For this review, take the finished solid that the model builds, in its own axes (mm). Face numbers are marked on the shaded views. Give positions to 0.01 mm unless a question says otherwise; leave off trailing zeros.
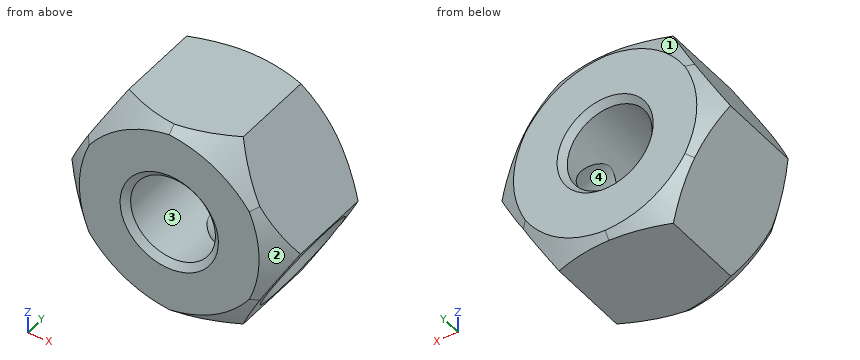
from build123d import *
from OCP.BRepFilletAPI import BRepFilletAPI_MakeChamfer

# Parameters (mm, degrees)
SKETCH1_R           = 1.5
BOSS_EXTRUDE1_DEPTH = 4.5
CHAMFER1_SIZE       = 0.2
CHAMFER1_SIZE2      = 0.238350719
SKETCH2_R           = 1.4
CUT_EXTRUDE1_DEPTH  = 3
CHAMFER2_SIZE       = 0.4
CHAMFER2_SIZE_2     = 0.476701437
FILLET1_R           = 5.5


with BuildPart() as part:
    # Sketch1 → Boss-Extrude1 (new body)
    with BuildSketch(Plane(origin=(0, 0, 0), x_dir=(1, 0, 0), z_dir=(0, 1, 0))):
        Polygon((4.041451884, 0), (2.020725942, 3.5), (-2.020725942, 3.5), (-4.041451884, 0), (-2.020725942, -3.5), (2.020725942, -3.5), align=None)
        with Locations(Location((0, 0, 0), (0, 0, 270))):
            Circle(SKETCH1_R, mode=Mode.SUBTRACT)
    extrude(amount=BOSS_EXTRUDE1_DEPTH)

    # Chamfer1: one chamfer whose edges measure the first distance from different faces: ONE call of the kernel's chamfer builder (chamfer() names one face for all edges)
    chamfer1_edges_1 = [part.edges().sort_by_distance(p)[0] for p in [
        (0, 4.5, -3.5),
    ]]
    chamfer1_side_1 = [part.faces().sort_by_distance(p)[0] for p in [
        (0, 2.25, -3.5),
    ]]
    chamfer1_edges_2 = [part.edges().sort_by_distance(p)[0] for p in [
        (-3.031088913, 4.5, -1.75),
    ]]
    chamfer1_side_2 = [part.faces().sort_by_distance(p)[0] for p in [
        (-3.031088913, 2.25, -1.75),
    ]]
    chamfer1_edges_3 = [part.edges().sort_by_distance(p)[0] for p in [
        (-3.031088913, 4.5, 1.75),
    ]]
    chamfer1_side_3 = [part.faces().sort_by_distance(p)[0] for p in [
        (-3.031088913, 2.25, 1.75),
    ]]
    chamfer1_edges_4 = [part.edges().sort_by_distance(p)[0] for p in [
        (0, 0, -1.5),
    ]]
    chamfer1_side_4 = [part.faces().sort_by_distance(p)[0] for p in [
        (0, 2.25, -1.5),
    ]]
    chamfer1_edges_5 = [part.edges().sort_by_distance(p)[0] for p in [
        (0, 4.5, -1.5),
    ]]
    chamfer1_side_5 = [part.faces().sort_by_distance(p)[0] for p in [
        (2.938487617, 4.5, -1.696536617),
    ]]
    chamfer1_edges_6 = [part.edges().sort_by_distance(p)[0] for p in [
        (0, 4.5, 3.5),
    ]]
    chamfer1_side_6 = [part.faces().sort_by_distance(p)[0] for p in [
        (0, 2.25, 3.5),
    ]]
    chamfer1_edges_7 = [part.edges().sort_by_distance(p)[0] for p in [
        (3.031088913, 4.5, 1.75),
    ]]
    chamfer1_side_7 = [part.faces().sort_by_distance(p)[0] for p in [
        (3.031088913, 2.25, 1.75),
    ]]
    chamfer1_edges_8 = [part.edges().sort_by_distance(p)[0] for p in [
        (0, 0, 3.5),
        (-3.031088913, 0, 1.75),
        (-3.031088913, 0, -1.75),
        (0, 0, -3.5),
        (3.031088913, 0, -1.75),
        (3.031088913, 0, 1.75),
    ]]
    chamfer1_side_8 = [part.faces().sort_by_distance(p)[0] for p in [
        (2.938487617, 0, -1.696536617),
    ]]
    chamfer1_edges_9 = [part.edges().sort_by_distance(p)[0] for p in [
        (3.031088913, 4.5, -1.75),
    ]]
    chamfer1_side_9 = [part.faces().sort_by_distance(p)[0] for p in [
        (3.031088913, 2.25, -1.75),
    ]]
    chamfer1 = BRepFilletAPI_MakeChamfer(part.part.solid().wrapped)
    for e in chamfer1_edges_1:
        chamfer1.Add(CHAMFER1_SIZE, CHAMFER1_SIZE2, e.wrapped, chamfer1_side_1[0].wrapped)  # the first distance lies on this face
    for e in chamfer1_edges_2:
        chamfer1.Add(CHAMFER1_SIZE, CHAMFER1_SIZE2, e.wrapped, chamfer1_side_2[0].wrapped)  # the first distance lies on this face
    for e in chamfer1_edges_3:
        chamfer1.Add(CHAMFER1_SIZE, CHAMFER1_SIZE2, e.wrapped, chamfer1_side_3[0].wrapped)  # the first distance lies on this face
    for e in chamfer1_edges_4:
        chamfer1.Add(CHAMFER1_SIZE, CHAMFER1_SIZE2, e.wrapped, chamfer1_side_4[0].wrapped)  # the first distance lies on this face
    for e in chamfer1_edges_5:
        chamfer1.Add(CHAMFER1_SIZE, CHAMFER1_SIZE2, e.wrapped, chamfer1_side_5[0].wrapped)  # the first distance lies on this face
    for e in chamfer1_edges_6:
        chamfer1.Add(CHAMFER1_SIZE, CHAMFER1_SIZE2, e.wrapped, chamfer1_side_6[0].wrapped)  # the first distance lies on this face
    for e in chamfer1_edges_7:
        chamfer1.Add(CHAMFER1_SIZE, CHAMFER1_SIZE2, e.wrapped, chamfer1_side_7[0].wrapped)  # the first distance lies on this face
    for e in chamfer1_edges_8:
        chamfer1.Add(CHAMFER1_SIZE, CHAMFER1_SIZE2, e.wrapped, chamfer1_side_8[0].wrapped)  # the first distance lies on this face
    for e in chamfer1_edges_9:
        chamfer1.Add(CHAMFER1_SIZE, CHAMFER1_SIZE2, e.wrapped, chamfer1_side_9[0].wrapped)  # the first distance lies on this face
    add(Compound.cast(chamfer1.Shape()), mode=Mode.REPLACE)

    # Sketch2 → Cut-Extrude1 (cut)
    with BuildSketch(Plane(origin=(3.031088913, 0, -1.75), x_dir=(-0.5, 0, -0.8660254037844386), z_dir=(0.8660254037844387, 0, -0.5000000000000001))):
        with Locations((0, 2.519175359)):
            Circle(SKETCH2_R)
    extrude(amount=-CUT_EXTRUDE1_DEPTH, mode=Mode.SUBTRACT)

    # Chamfer2
    # the kernel refuses this chamfer: 0.476701437, 0.4 mm, written as the material it takes off along each edge
    with BuildSketch(Plane(origin=(3.031088913, 2.519175359, -1.75), x_dir=(-0.5000000000000001, 0, -0.8660254037844386), z_dir=(0, -1, 0))) as chamfer2_piece_1:
        Polygon((1.4 + CHAMFER2_SIZE, 0), (1.4, -CHAMFER2_SIZE_2), (1.4, 0), align=None)
    revolve(axis=Axis((3.031088913, 2.519175359, -1.75), (0.8660254037844387, 0, -0.5000000000000001)), mode=Mode.SUBTRACT)

    # Fillet1
    # the kernel refuses this fillet: 5.5 mm, written as the material it takes off along each edge
    with BuildSketch(Plane(origin=(0.15679227, -4.094610415, 0), x_dir=(0.2750801350308494, 0.26652756240167075, 0.9237391286459793), z_dir=(-0.6958540455341976, 0.7181832268395656, -6.118874277733391e-15)), Plane(origin=(-0.15679227, -4.094610415, 0), x_dir=(-0.2750801350308542, 0.2665275624016659, -0.9237391286459793), z_dir=(0.6958540455341957, 0.7181832268395675, 0)), Plane(origin=(-0.078396135, -4.094610415, -0.135786089), x_dir=(0.6624414843616913, 0.266527562401667, -0.7000959493361638), z_dir=(0.347927022767099, 0.7181832268395667, 0.6026272807587874)), Plane(origin=(0.078396135, -4.094610415, -0.135786089), x_dir=(0.937521619392547, 0.2665275624016655, 0.2236431793098164), z_dir=(-0.3479270227670974, 0.718183226839567, 0.6026272807587876))) as fillet1_piece_1:
        with BuildLine():
            CenterArc((FILLET1_R * 0.414643279343, FILLET1_R), FILLET1_R, 224.957975764, 45.042024236)
            Line((-FILLET1_R * 0.292981947048, FILLET1_R * 0.293412044417), (0, 0))
            Line((0, 0), (FILLET1_R * 0.414643279343, 0))
        make_face()
    extrude(amount=11.734570278, mode=Mode.SUBTRACT)
    with BuildSketch(Plane(origin=(0.078396135, -4.094610415, 0.135786089), x_dir=(0.9375216193925491, 0.26652756240166126, -0.22364317930981242), z_dir=(-0.3479270227670917, 0.7181832268395687, -0.602627280758789)), Plane(origin=(-0.078396135, -4.094610415, 0.135786089), x_dir=(0.6624414843616925, 0.2665275624016671, 0.7000959493361628), z_dir=(0.3479270227670974, 0.718183226839567, -0.6026272807587876))) as fillet1_piece_2:
        with BuildLine():
            CenterArc((FILLET1_R * 0.414643279343, -FILLET1_R), FILLET1_R, 90, 45.042024236)
            Line((-FILLET1_R * 0.292981947048, -FILLET1_R * 0.293412044417), (0, 0))
            Line((0, 0), (FILLET1_R * 0.414643279343, 0))
        make_face()
    extrude(amount=11.734570278, mode=Mode.SUBTRACT)
    with BuildSketch(Plane(origin=(3.908343828, 1.556605641, -6.769450083), x_dir=(0.7256118681846667, -0.25999585509227957, 0.6370946335391565), z_dir=(-0.40448174665200637, 0.5878588831525535, 0.7005829359354784)), Plane(origin=(-3.908343828, 1.556605641, -6.769450083), x_dir=(0.9145460713519834, -0.25999585509227496, -0.3098509943658236), z_dir=(0.4044817466520002, 0.5878588831525553, 0.7005829359354805)), Plane(origin=(-7.816687655, 1.556605641, 0), x_dir=(0.18893420316732476, -0.2599958550922833, -0.9469456279049819), z_dir=(0.8089634933040146, 0.5878588831525519, 7.47827698098615e-15))) as fillet1_piece_3:
        with BuildLine():
            CenterArc((FILLET1_R * 0.339400484434, -FILLET1_R), FILLET1_R, 90, 37.494474502)
            Line((-FILLET1_R * 0.269284432231, -FILLET1_R * 0.206587955583), (0, 0))
            Line((0, 0), (FILLET1_R * 0.339400484434, 0))
        make_face()
    extrude(amount=9.673731027, mode=Mode.SUBTRACT)
    with BuildSketch(Plane(origin=(7.816687655, 1.556605641, 0), x_dir=(-0.18893420316731485, -0.2599958550922788, -0.946945627904985), z_dir=(-0.8089634933040131, 0.587858883152554, 0)), Plane(origin=(3.908343828, 1.556605641, 6.769450083), x_dir=(0.7256118681846656, -0.25999585509228007, -0.6370946335391575), z_dir=(-0.40448174665200737, 0.5878588831525533, -0.7005829359354782)), Plane(origin=(-3.908343828, 1.556605641, 6.769450083), x_dir=(0.9145460713519806, -0.25999585509227907, 0.30985099436582814), z_dir=(0.4044817466520063, 0.5878588831525535, -0.7005829359354784))) as fillet1_piece_4:
        with BuildLine():
            CenterArc((FILLET1_R * 0.339400484434, FILLET1_R), FILLET1_R, 232.505525498, 37.494474502)
            Line((-FILLET1_R * 0.269284432231, FILLET1_R * 0.206587955583), (0, 0))
            Line((0, 0), (FILLET1_R * 0.339400484434, 0))
        make_face()
    extrude(amount=9.673731027, mode=Mode.SUBTRACT)


solid = part.part
1) To check wall thickness, follow line 1 (Z direction, x = 0, y = 2); line 2 (Z direction, x = 1, y = 1); line 3 (X direction, y = 3.95, z = 0.5). State the ranges of each line that lie inside material, in increasing order.
Answer sheet:
line 1: z = -3.5 to -1.5, 1.5 to 3.5
line 2: z = -3.5 to -1.12, 1.12 to 3.5
line 3: x = -3.75 to -1.41, 1.41 to 3.75
2) Clearance check with a flat-ended pin moving along its axis: pin 1 (1.5 mm diameter, centred on y = 2.5, z = -2, fed in from +X). State where the tip first meets the part, or that it passes through.
Answer sheet:
pin 1: stops at x = 1.93
3) Draft analysis for pull direction Z (two halves, no side actions). For the marked faces 1, 2, 3 and 4, state which applies: +Z half, -Z half, draft (parallel to the pull), parting line (faces both ways), or undercut.
Answer sheet:
face 1: +Z half
face 2: parting line
face 3: undercut
face 4: undercut
